```python
from build123d import *

# Parameters (mm, degrees)
F0_R     = 9.525
F1_DEPTH = 4.064
F2_R     = 4.064
F3_DEPTH = 34.925
F4_R     = 4.064
F5_DEPTH = 34.925
F6_R     = 0.508
F7_DEPTH = 5.08


with BuildPart() as f1:
    # F0 (on Top) → F1 (new body, symmetric)
    with BuildSketch(Plane.XY):
        Circle(F0_R)
    extrude(amount=F1_DEPTH, both=True)

    # F2 (on Right) → F3 (join, symmetric)
    with BuildSketch(Plane.YZ):
        Circle(F2_R)
    extrude(amount=F3_DEPTH, both=True)

    # F4 (on Front) → F5 (join, symmetric)
    with BuildSketch(Plane.XZ):
        Circle(F4_R)
    extrude(amount=F5_DEPTH, both=True)

    # F6 (on face) → F7 (cut)
    with BuildSketch(Plane.XY.offset(4.064)):
        Circle(F6_R)
    extrude(amount=-F7_DEPTH, mode=Mode.SUBTRACT)


solid = f1.part
```
Design review of the part built by this model. Coordinates are the model's own, in mm. A direction names the side the tool comes from. Coordinates: 2 decimals unless noted, no trailing zeros. Write each loop counter-clockwise with the first axis right and the second up, starting at its lowest first coordinate (ties: lowest second). Pieces come first, ordered by that corner, then holes. Notation, with made-up numbers: M 33.25,18 L 53.25,18 A29 cw 53.25,53 Z; hole C 7.25,24.25 d11. An arc over 180 degrees is marked long. Answer as a JSON object with one key per item and string values.
Item 1: Wall thickness on probe 1 along Y at (x, z) = (0, 1.65) (3 decimals); probe 2 along Y at (x, z) = (29.5, 0): over which ranges is each line inside the solid? List them lowest first.
Outcome:
{"probe 1": "-34.925 to -0.508, 0.508 to 34.925", "probe 2": "-4.06 to 4.06"}
Item 2: Insertion check: pin 1 Ø1.5 at (x, z) = (-25, -2.5) entering from +Y; pin 2 Ø4 at (y, z) = (18.5, -2.5) entering from -X. Each pin has a flat end and moves straight along its axis. Give the tip position at first contact, or say it passes through.
Outcome:
{"pin 1": "y = 3.67", "pin 2": "x = -4.03"}
Item 3: Draft analysis for pull direction Y (two halves, no side actions). For faces 4 (the cylindrical face through (-21.586, -0.881, -3.967)), 5 (the cylindrical face through (-6.81, -6.66, 0.06)), 6 (the cylindrical face through (-6.66, 6.81, 0.06)), 7 (the cylindrical face through (-0.881, -21.954, -3.967)), state which applies: pulls with the +Y half, pulls with the -Y half, needs draft (parallel to the pull), parting line crosses it, or undercut.
Outcome:
{"face 4": "parting line crosses it", "face 5": "pulls with the -Y half", "face 6": "pulls with the +Y half", "face 7": "needs draft"}
Item 4: Add section C-C, the plane x = 11.5. Give the boundary of the cut face in (y, z), and give its area (3 significant figures).
Outcome:
{"outline": "C 0,0 d8.13", "area": "51.9 mm²"}
Item 5: Add section B-B, the plane y = 3. Give the boundary of the cut face in (x, z) (3 decimals), and give its area (3 significant figures).
Outcome:
{"outline": "M -34.925,-2.742 L -9.04,-2.742 L -9.04,-4.064 L 9.04,-4.064 L 9.04,-2.742 L 34.925,-2.742 L 34.925,2.742 L 9.04,2.742 L 9.04,4.064 L -9.04,4.064 L -9.04,2.742 L -34.925,2.742 Z", "area": "431 mm²"}
Item 6: Machinability: for faces 1 (the flat face through (34.925, 0, 0)), 2 (the cylindrical face through (21.954, -0.881, -3.967)), 3 (the cylindrical face through (-0.881, 21.586, -3.967)), which of the approach directions +Z, -Z, +X, -X, +Y, -Y give a long, thin tool a straight path to every point of the face, cutting with its end or side? Answer none if there is none.
Outcome:
{"face 1": "+Z, -Z, +X, +Y, -Y", "face 2": "+X", "face 3": "+Y"}
